Source: CAD feature listing. Evaluate the final solid. Frame: model axes, mm. Round coordinates to 2 decimals unless told otherwise and drop trailing zeros. Order: outer loops, then holes, each group sorted by start corner. A loop starts at its lowest first (then second) coordinate and runs counter-clockwise, first axis right, second up. Notation, with made-up numbers: M -8,65 L 8,65 A18 ccw 8,100 Z; hole C 80,-6 d1. An arc over 180 degrees is marked long. Use one line per item in the form item = value. Start each with the question number.
Q1. Section C-C (z = -38.5). Return the cut outline in (x, y).
Q2. Material intervals for probe 1 along Z at (x, y) = (0, 2.05); probe 2 along Z at (x, y) = (-19.5, 0.3); probe 3 along X at (y, z) = (4.5, -6.5), sorted ascending.
Q3. Section B-B (z = 0). Return the cut outline in (x, y).
Q4. Section D-D (x = 36.5). Return the cut outline in (y, z).
Q5. Contact query for flat-ended pins moving along their axis: pin 1 (1 mm diameter, centred on y = 4, z = -24, fed in from -X); pin 2 (1 mm diameter, centred on y = 1, z = 15, fed in from -X); pin 3 (1.4 mm diameter, centred on y = 1.5, z = 2, fed in from +X). Output: stop coordinate, or through.
Q6. Section A-A (x = 0). Return the cut outline in (y, z).
from build123d import *

# Parameters (mm, degrees)
BOSS_EXTRUDE1_DEPTH = 4.7625


with BuildPart() as part:
    # Sketch1 → Boss-Extrude1 (new body)
    with BuildSketch(Plane(origin=(0, 0, 0), x_dir=(1, 0, 0), z_dir=(0, 1, 0))):
        with BuildLine():
            ThreePointArc((-33.928372628, 33.36566521), (-35.574336427, 20.538852712), (-45.8597, 12.7))
            Line((-45.8597, 12.7), (-45.8597, 5.950469261))
            ThreePointArc((-45.8597, 5.950469261), (-40.084375, 0), (-45.8597, -5.950469261))
            Line((-45.8597, -5.950469261), (-45.8597, -12.7))
            ThreePointArc((-45.8597, -12.7), (-35.574336427, -20.538852712), (-33.928372628, -33.36566521))
            Line((-33.928372628, -33.36566521), (-28.083107544, -36.740430579))
            ThreePointArc((-28.083107544, -36.740430579), (-20.0421875, -34.714087045), (-17.776592456, -42.69089984))
            Line((-17.776592456, -42.69089984), (-11.931327372, -46.06566521))
            ThreePointArc((-11.931327372, -46.06566521), (0, -41.077705425), (11.931327372, -46.06566521))
            Line((11.931327372, -46.06566521), (17.776592456, -42.69089984))
            ThreePointArc((17.776592456, -42.69089984), (20.0421875, -34.714087045), (28.083107544, -36.740430579))
            Line((28.083107544, -36.740430579), (33.928372628, -33.36566521))
            ThreePointArc((33.928372628, -33.36566521), (35.574336427, -20.538852712), (45.8597, -12.7))
            Line((45.8597, -12.7), (45.8597, -5.950469261))
            ThreePointArc((45.8597, -5.950469261), (40.084375, 0), (45.8597, 5.950469261))
            Line((45.8597, 5.950469261), (45.8597, 12.7))
            ThreePointArc((45.8597, 12.7), (35.574336427, 20.538852712), (33.928372628, 33.36566521))
            Line((33.928372628, 33.36566521), (28.083107544, 36.740430579))
            ThreePointArc((28.083107544, 36.740430579), (20.0421875, 34.714087045), (17.776592456, 42.69089984))
            Line((17.776592456, 42.69089984), (11.931327372, 46.06566521))
            ThreePointArc((11.931327372, 46.06566521), (0, 41.077705425), (-11.931327372, 46.06566521))
            Line((-11.931327372, 46.06566521), (-17.776592456, 42.69089984))
            ThreePointArc((-17.776592456, 42.69089984), (-20.0421875, 34.714087045), (-28.083107544, 36.740430579))
            Line((-28.083107544, 36.740430579), (-33.928372628, 33.36566521))
        make_face()
        with BuildLine():
            Line((1.374815329, 20.455395717), (17.027484671, 11.418322859))
            ThreePointArc((17.027484671, 11.418322859), (18.813175234, 12.157980108), (19.9898, 10.624572859))
            ThreePointArc((19.9898, 10.624572859), (19.524832015, 9.502040844), (18.4023, 9.037072859))
            Line((18.4023, 9.037072859), (18.4023, -9.037072859))
            ThreePointArc((18.4023, -9.037072859), (19.524832015, -9.502040844), (19.9898, -10.624572859))
            ThreePointArc((19.9898, -10.624572859), (18.813175234, -12.157980108), (17.027484671, -11.418322859))
            Line((17.027484671, -11.418322859), (1.374815329, -20.455395717))
            ThreePointArc((1.374815329, -20.455395717), (1.533407249, -20.838270483), (1.5875, -21.249145717))
            ThreePointArc((1.5875, -21.249145717), (-0.410875234, -22.782552967), (-1.374815329, -20.455395717))
            Line((-1.374815329, -20.455395717), (-17.027484671, -11.418322859))
            ThreePointArc((-17.027484671, -11.418322859), (-19.777115329, -11.418322859), (-18.4023, -9.037072859))
            Line((-18.4023, -9.037072859), (-18.4023, 9.037072859))
            ThreePointArc((-18.4023, 9.037072859), (-19.777115329, 11.418322859), (-17.027484671, 11.418322859))
            Line((-17.027484671, 11.418322859), (-1.374815329, 20.455395717))
            ThreePointArc((-1.374815329, 20.455395717), (-0.410875234, 22.782552967), (1.5875, 21.249145717))
            ThreePointArc((1.5875, 21.249145717), (1.533407249, 20.838270483), (1.374815329, 20.455395717))
        make_face(mode=Mode.SUBTRACT)
    extrude(amount=BOSS_EXTRUDE1_DEPTH)


solid = part.part
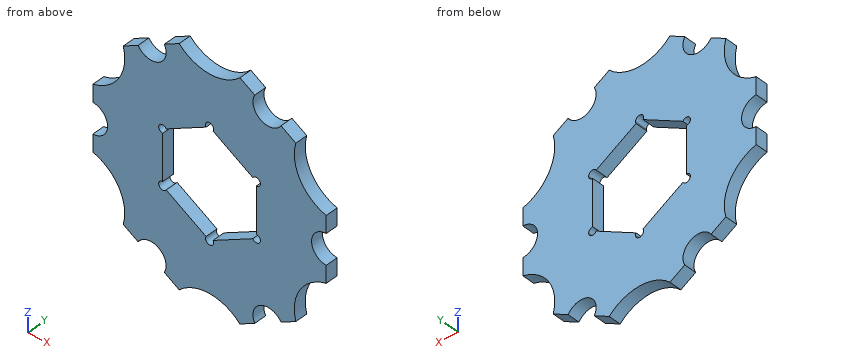
Results list:
q1.outline = M -17.23,0 L 17.23,0 L 17.23,4.76 L -17.23,4.76 Z
q2.probe_1 = -41.08 to -22.84, 22.84 to 41.08
q2.probe_2 = -35.07 to -11.77, -9.48 to 9.48, 11.77 to 35.07
q2.probe_3 = -45.86 to -18.4, 18.4 to 45.86
q3.outline = M -40.08,0 L -18.4,0 L -18.4,4.76 L -40.08,4.76 Z; M 18.4,0 L 40.08,0 L 40.08,4.76 L 18.4,4.76 Z
q4.outline = M 0,-19.11 L 4.76,-19.11 L 4.76,19.11 L 0,19.11 Z
q5.pin_1 = -34.23
q5.pin_2 = -41.54
q5.pin_3 = 40.73
q6.outline = M 0,-41.08 L 4.76,-41.08 L 4.76,-22.84 L 0,-22.84 Z; M 0,22.84 L 4.76,22.84 L 4.76,41.08 L 0,41.08 Z
